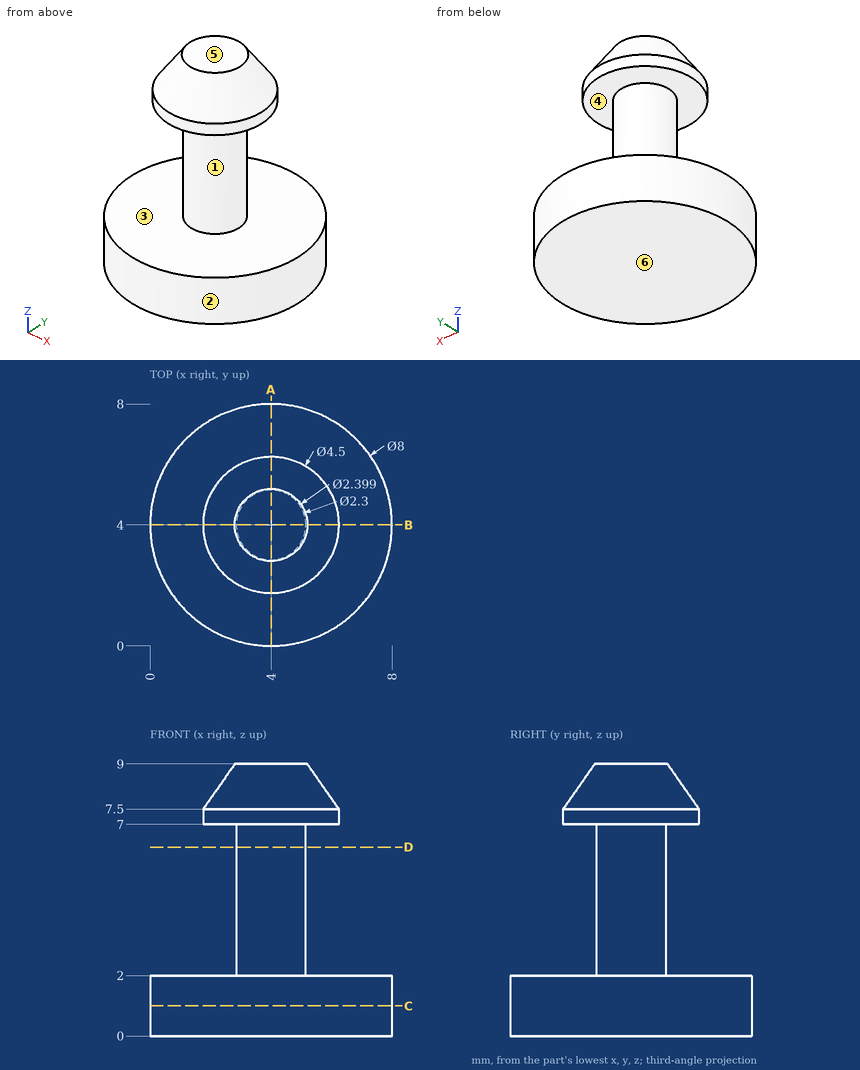
Check sheet for the drawn part. Datum: minimum x, y, z corner. Units: mm. A direction names the side the tool comes from. Give positions to 0.01 mm unless a question says otherwise; leave off trailing zeros. Order: outer loops, then holes, each group sorted by start corner. A loop starts at its lowest first (then second) coordinate and runs counter-clockwise, first axis right, second up. Notation, with made-up numbers: (-39.5, -29.75) -> (-17.5, -29.75) arc R24 cw to (-17.5, -6.75) -> close; hole circle Ø5 at (78.5, -15). An arc over 180 degrees is marked (long way). Return JSON: item names as keys, results as strings.
1. Cross-section at A-A, the plane x = 4. Record the cut outline in (y, z).
From the geometry:
{"outline": "(0, 0) -> (8, 0) -> (8, 2) -> (5.15, 2) -> (5.15, 7) -> (6.25, 7) -> (6.25, 7.5) -> (5.2, 9) -> (2.8, 9) -> (1.75, 7.5) -> (1.75, 7) -> (2.85, 7) -> (2.85, 2) -> (0, 2) -> close"}
2. Mould release check, pull along Z, two halves, no side actions. Record for the marked faces 3, 4, 5 and 6: +Z half, -Z half, draft (parallel to the pull), parting line (faces both ways), or undercut.
From the geometry:
{"face 3": "undercut", "face 4": "undercut", "face 5": "+Z half", "face 6": "-Z half"}
3. Material ranges on probe 1 along Z at (x, y) = (4.75, 2.25) (1 decimal); probe 2 along Z at (x, y) = (2.25, 5.75); probe 3 along Z at (x, y) = (6, 3.25) (1 decimal), recorded low to high. Write a range as [from, to].
From the geometry:
{"probe 1": "[0, 2], [7, 8]", "probe 2": "[0, 2]", "probe 3": "[0, 2], [7, 7.7]"}
4. Set-up check for the marked faces 1 and 2: record each of +Z, -Z, +X, -X, +Y, -Y from which the full face is reachable in a straight line by a thin tool's end or side.
From the geometry:
{"face 1": "none", "face 2": "+Z, -Z"}
5. Cross-section at C-C, the plane z = 1. Record the cut outline in (x, y).
From the geometry:
{"outline": "circle Ø8 at (4, 4)"}
6. Cross-section at D-D, the plane z = 6.25. Record the cut outline in (x, y).
From the geometry:
{"outline": "circle Ø2.3 at (4, 4)"}
7. Go/stop test with flat-tipped pins: P1, Ø1.5, axis at x = 7, y = 5.5, coming from the +Z side; P2, Ø4, axis at x = 6.5, y = 7, coming from the +Z side; P3, Ø3, axis at x = 7, z = 6, coming from the -Y side (1 decimal). Record where each tip stops, or that it passes through.
From the geometry:
{"P1": "z = 2", "P2": "z = 7.99", "P3": "y = 2.8"}
